```python
from build123d import *

# Parameters (mm, degrees)
SKETCH_1_R      = 62.5
SKETCH_1_R_2    = 2
SKETCH_1_R_3    = 1.5
SKETCH_1_R_4    = 6.5
SKETCH_1_R_5    = 0.75
EXTRUDE_1_DEPTH = 2


with BuildPart() as part:
    # 草图1 → 凸台-拉伸1 (new body)
    with BuildSketch(Plane.XY):
        Circle(SKETCH_1_R)
        with Locations((0, -20)):
            Circle(SKETCH_1_R_2, mode=Mode.SUBTRACT)
        with Locations((0, -59)):
            Circle(SKETCH_1_R_3, mode=Mode.SUBTRACT)
        with Locations((-20, 0)):
            Circle(SKETCH_1_R_2, mode=Mode.SUBTRACT)
        with Locations((0, 20)):
            Circle(SKETCH_1_R_2, mode=Mode.SUBTRACT)
        with Locations((20, 0)):
            Circle(SKETCH_1_R_2, mode=Mode.SUBTRACT)
        with Locations((-31.89780823, -49.633958437)):
            Circle(SKETCH_1_R_3, mode=Mode.SUBTRACT)
        with Locations((-53.668287726, -24.509485767)):
            Circle(SKETCH_1_R_3, mode=Mode.SUBTRACT)
        with Locations((-58.399465071, 8.396575458)):
            Circle(SKETCH_1_R_3, mode=Mode.SUBTRACT)
        with Locations((-44.589224887, 38.636783303)):
            Circle(SKETCH_1_R_3, mode=Mode.SUBTRACT)
        with Locations((-16.622220854, 56.610085443)):
            Circle(SKETCH_1_R_3, mode=Mode.SUBTRACT)
        with Locations((16.622220854, 56.610085443)):
            Circle(SKETCH_1_R_3, mode=Mode.SUBTRACT)
        with Locations((44.589224887, 38.636783303)):
            Circle(SKETCH_1_R_3, mode=Mode.SUBTRACT)
        with Locations((58.399465071, 8.396575458)):
            Circle(SKETCH_1_R_3, mode=Mode.SUBTRACT)
        with Locations((53.668287726, -24.509485767)):
            Circle(SKETCH_1_R_3, mode=Mode.SUBTRACT)
        with Locations((31.89780823, -49.633958437)):
            Circle(SKETCH_1_R_3, mode=Mode.SUBTRACT)
        Circle(SKETCH_1_R_4, mode=Mode.SUBTRACT)
        with Locations((-7.498513861, -7.498513861)):
            Circle(SKETCH_1_R_5, mode=Mode.SUBTRACT)
        with Locations((-7.498513861, 7.498513861)):
            Circle(SKETCH_1_R_5, mode=Mode.SUBTRACT)
        with Locations((7.498513861, 7.498513861)):
            Circle(SKETCH_1_R_5, mode=Mode.SUBTRACT)
        with Locations((7.498513861, -7.498513861)):
            Circle(SKETCH_1_R_5, mode=Mode.SUBTRACT)
        with BuildLine():
            Line((-46.475800154, 4), (-27.110883423, 4))
            ThreePointArc((-27.110883423, 4), (-25.273766116, 4.628291755), (-24.206145914, 6.25))
            ThreePointArc((-24.206145914, 6.25), (-17.67766953, 17.67766953), (-6.25, 24.206145914))
            ThreePointArc((-6.25, 24.206145914), (-4.628291755, 25.273766116), (-4, 27.110883423))
            Line((-4, 27.110883423), (-4, 46.475800154))
            ThreePointArc((-4, 46.475800154), (-5.043015781, 48.749610341), (-7.446808511, 49.44234059))
            ThreePointArc((-7.446808511, 49.44234059), (-35.355339059, 35.355339059), (-49.44234059, 7.446808511))
            ThreePointArc((-49.44234059, 7.446808511), (-48.749610341, 5.043015781), (-46.475800154, 4))
        make_face(mode=Mode.SUBTRACT)
        with BuildLine():
            Line((4, 46.475800154), (4, 27.110883423))
            ThreePointArc((4, 27.110883423), (4.628291755, 25.273766116), (6.25, 24.206145914))
            ThreePointArc((6.25, 24.206145914), (17.67766953, 17.67766953), (24.206145914, 6.25))
            ThreePointArc((24.206145914, 6.25), (25.273766116, 4.628291755), (27.110883423, 4))
            Line((27.110883423, 4), (46.475800154, 4))
            ThreePointArc((46.475800154, 4), (48.749610341, 5.043015781), (49.44234059, 7.446808511))
            ThreePointArc((49.44234059, 7.446808511), (35.355339059, 35.355339059), (7.446808511, 49.44234059))
            ThreePointArc((7.446808511, 49.44234059), (5.043015781, 48.749610341), (4, 46.475800154))
        make_face(mode=Mode.SUBTRACT)
        with BuildLine():
            Line((-27.110883423, -4), (-46.475800154, -4))
            ThreePointArc((-46.475800154, -4), (-48.749610341, -5.043015781), (-49.44234059, -7.446808511))
            ThreePointArc((-49.44234059, -7.446808511), (-35.355339059, -35.355339059), (-7.446808511, -49.44234059))
            ThreePointArc((-7.446808511, -49.44234059), (-5.043015781, -48.749610341), (-4, -46.475800154))
            Line((-4, -46.475800154), (-4, -27.110883423))
            ThreePointArc((-4, -27.110883423), (-4.628291755, -25.273766116), (-6.25, -24.206145914))
            ThreePointArc((-6.25, -24.206145914), (-17.67766953, -17.67766953), (-24.206145914, -6.25))
            ThreePointArc((-24.206145914, -6.25), (-25.273766116, -4.628291755), (-27.110883423, -4))
        make_face(mode=Mode.SUBTRACT)
        with BuildLine():
            Line((46.475800154, -4), (27.110883423, -4))
            ThreePointArc((27.110883423, -4), (25.273766116, -4.628291755), (24.206145914, -6.25))
            ThreePointArc((24.206145914, -6.25), (17.67766953, -17.67766953), (6.25, -24.206145914))
            ThreePointArc((6.25, -24.206145914), (4.628291755, -25.273766116), (4, -27.110883423))
            Line((4, -27.110883423), (4, -46.475800154))
            ThreePointArc((4, -46.475800154), (5.043015781, -48.749610341), (7.446808511, -49.44234059))
            ThreePointArc((7.446808511, -49.44234059), (35.355339059, -35.355339059), (49.44234059, -7.446808511))
            ThreePointArc((49.44234059, -7.446808511), (48.749610341, -5.043015781), (46.475800154, -4))
        make_face(mode=Mode.SUBTRACT)
    extrude(amount=EXTRUDE_1_DEPTH)


solid = part.part
```
Input: part model. Units: mm. Frame: model coordinates. A direction names the side the tool comes from. Coordinates: 2 decimals unless noted, no trailing zeros. Write each loop counter-clockwise with the first axis right and the second up, starting at its lowest first coordinate (ties: lowest second). Pieces come first, ordered by that corner, then holes.
1) Mould query, pull axis X, two halves, no side actions, for faces 1 (the cylindrical face through (-62.44, 2.75, 0.99)), 2 (the cylindrical face through (-17.809, 17.545, 0.986)), 3 (the flat face through (-1, -13, 0)). Classes: pulls with the +X half, pulls with the -X half, needs draft (parallel to the pull), parting line crosses it, or undercut.
2) Section C-C on y = -59. Output: boundary loops of the cut face in (x, z), and give its area (3 significant figures).
3) Pin query (flat end, axial travel): pin 1 Ø2.5 at (x, y) = (-44.59, 38.64) entering from -Z; pin 2 Ø1 at (y, z) = (15, 1) entering from +X; pin 3 Ø1 at (y, z) = (37, 1) entering from +X. Return the tip coordinate at first contact, or that it passes through.
4) Material intervals for line 1 along Y through (x, z) = (0, 0.65); line 2 along X through (y, z) = (21, 0.55); line 3 along Y through (x, z) = (-10.5, 0.1), sorted ascending.
5) Section D-D on x = 40.5. Output: boundary loops of the cut face in (y, z).
6) Set-up query: faces 4 (the cylindrical face through (-5.02, 48.73, 0.99)), 5 (the flat face through (-1, -13, 2)). Return all of +Z, -Z, +X, -X, +Y, -Y with unobstructed straight access to the full face (end or side cutting, diameter ignored); none if empty.
7) Section A-A on x = 0. Output: boundary loops of the cut face in (y, z), and give its area (3 significant figures).
8) Section B-B on y = 0. Output: boundary loops of the cut face in (x, z), and give its area (3 significant figures).
Check result:
1. face 1: parting line crosses it
1. face 2: undercut
1. face 3: needs draft
2. outline: (-20.62, 0) - (-1.5, 0) - (-1.5, 2) - (-20.62, 2) - close; (1.5, 0) - (20.62, 0) - (20.62, 2) - (1.5, 2) - close
2. area: 76.5 mm2
3. pin 1: passes through
3. pin 2: stops at x = 60.79
3. pin 3: stops at x = 50.73
4. line 1: y = -62.5 to -60.5, -57.5 to -22, -18 to -6.5, 6.5 to 18, 22 to 62.5
4. line 2: x = -58.87 to -45.38, -13.56 to -1.73, 1.73 to 13.56, 45.38 to 58.87
4. line 3: y = -61.61 to -48.89, -22.69 to 22.69, 48.89 to 61.61
5. outline: (-47.6, 0) - (-29.32, 0) - (-29.32, 2) - (-47.6, 2) - close; (-4, 0) - (4, 0) - (4, 2) - (-4, 2) - close; (29.32, 0) - (47.6, 0) - (47.6, 2) - (29.32, 2) - close
6. face 4: +Z, -Z
6. face 5: +Z, +X, -X, +Y, -Y
7. outline: (-62.5, 0) - (-60.5, 0) - (-60.5, 2) - (-62.5, 2) - close; (-57.5, 0) - (-22, 0) - (-22, 2) - (-57.5, 2) - close; (-18, 0) - (-6.5, 0) - (-6.5, 2) - (-18, 2) - close; (6.5, 0) - (18, 0) - (18, 2) - (6.5, 2) - close; (22, 0) - (62.5, 0) - (62.5, 2) - (22, 2) - close
7. area: 202 mm2
8. outline: (-62.5, 0) - (-22, 0) - (-22, 2) - (-62.5, 2) - close; (-18, 0) - (-6.5, 0) - (-6.5, 2) - (-18, 2) - close; (6.5, 0) - (18, 0) - (18, 2) - (6.5, 2) - close; (22, 0) - (62.5, 0) - (62.5, 2) - (22, 2) - close
8. area: 208 mm2
